```python
from build123d import *

# Parameters (mm, degrees)
SKETCH1_R           = 11.35
BOSS_EXTRUDE1_DEPTH = 18
SKETCH2_R           = 13.5
BOSS_EXTRUDE2_DEPTH = 3.2
FILLET1_R           = 3
SKETCH3_R           = 9.75
BOSS_EXTRUDE3_DEPTH = 3.72


with BuildPart() as part:
    # Sketch1 → Boss-Extrude1 (new body)
    with BuildSketch(Plane(origin=(0, 0, 0), x_dir=(1, 0, 0), z_dir=(0, 1, 0))):
        with Locations(Location((0, 0, 0), (0, 0, 270))):
            Circle(SKETCH1_R)
    extrude(amount=-BOSS_EXTRUDE1_DEPTH)

    # Sketch2 → Boss-Extrude2 (add)
    with BuildSketch(Plane(origin=(0, 0, 0), x_dir=(1, 0, 0), z_dir=(0, 1, 0))):
        with Locations(Location((0, 0, 0), (0, 0, 270))):
            Circle(SKETCH2_R)
    extrude(amount=BOSS_EXTRUDE2_DEPTH)

    # Fillet1
    fillet1_edges = [part.edges().sort_by_distance(p)[0] for p in [
        (0, 3.2, -13.5),
    ]]
    fillet(fillet1_edges, radius=FILLET1_R)

    # Sketch3 → Boss-Extrude3 (add)
    with BuildSketch(Plane(origin=(0, 3.2, 0), x_dir=(1, 0, 0), z_dir=(0, 1, 0))):
        with Locations(Location((0, 0, 0), (0, 0, 270))):
            Circle(SKETCH3_R)
    extrude(amount=BOSS_EXTRUDE3_DEPTH)


solid = part.part
```
CAD build for the part. Positions are in the model's coordinates, mm. A direction names the side the tool comes from. Round coordinates to 2 decimals unless told otherwise and drop trailing zeros. Loops run counter-clockwise (first coordinate to the right, second up) from the corner with the lowest first, then second, coordinate; pieces in that order, holes last. Notation, with made-up numbers: M 83,37.5 L 132,37.5 A29 cw 132,73.5 Z; hole C 23.25,10.5 d5. An arc over 180 degrees is marked long. Return JSON: item names as keys, results as strings. Group by question number.
(1) Tool access for faces 1 (the flat face through (0, 6.92, 0)), 2 (the flat face through (11.1, 0, -3.1)), 3 (the flat face through (-8, 3.2, 6)): list every direction of +Z, -Z, +X, -X, +Y, -Y with a clear straight run to the whole face (end or side of a thin tool).
(2) Saw through at A-A, the plane z = 0. List the corners of the cut face in (x, y).
(3) Saw through at B-B, the plane x = 0. List the corners of the cut face in (y, z).
(4) Saw through at C-C, the plane y = -6. List the corners of the cut face in (x, z).
(5) Drop flat-ended pins along their axis: P1, Ø3, axis at x = -2, y = -11.5, coming from the -Z side; P2, Ø2, axis at y = -6, z = 8, coming from the -X side; P3, Ø6, axis at y = -14, z = 11, coming from the -X side. Give the stop position or say it passes through.
(6) Wall check: probe 1 along Y at (x, z) = (-2, 9.75); probe 2 along Z at (x, y) = (-1.75, -14); probe 3 along X at (y, z) = (-8, 3.75). Give the ranges that are in metal, low to high. Write a range as [from, to].
Answer list:
{
 "1": {"face 1": "+Z, -Z, +X, -X, +Y", "face 2": "-Y", "face 3": "+Y"},
 "2": {"outline": "M -13.5,0 L -11.35,0 L -11.35,-18 L 11.35,-18 L 11.35,0 L 13.5,0 L 13.5,0.2 A3 ccw 10.5,3.2 L 9.75,3.2 L 9.75,6.92 L -9.75,6.92 L -9.75,3.2 L -10.5,3.2 A3 ccw -13.5,0.2 Z"},
 "3": {"outline": "M -18,-11.35 L 0,-11.35 L 0,-13.5 L 0.2,-13.5 A3 ccw 3.2,-10.5 L 3.2,-9.75 L 6.92,-9.75 L 6.92,9.75 L 3.2,9.75 L 3.2,10.5 A3 ccw 0.2,13.5 L 0,13.5 L 0,11.35 L -18,11.35 Z"},
 "4": {"outline": "C 0,0 d22.7"},
 "5": {"P1": "z = -11.34", "P2": "x = -8.93", "P3": "x = -8.05"},
 "6": {"probe 1": "[-18, 3.2]", "probe 2": "[-11.21, 11.21]", "probe 3": "[-10.71, 10.71]"}
}
